Source: CAD feature listing. Evaluate the final solid. Frame: model axes, mm. A direction names the side the tool comes from. Round coordinates to 2 decimals unless told otherwise and drop trailing zeros. Order: outer loops, then holes, each group sorted by start corner. A loop starts at its lowest first (then second) coordinate and runs counter-clockwise, first axis right, second up. Notation, with made-up numbers: M 27.25,-34.75 L 63.25,-34.75 A18 ccw 63.25,-6.75 Z; hole C 55.5,-18.5 d8. An arc over 180 degrees is marked long. Answer in a Markdown table with one row per item. Add a question column.
```python
from build123d import *

# Parameters (mm, degrees)
F0_W     = 32
F0_H     = 19
F1_DEPTH = 4
F2_W     = 32
F2_H     = 4
F3_DEPTH = 16
F5_W     = 14
F5_H     = 6.1
F6_DEPTH = 25
F7_R     = 1.85
F8_DEPTH = 2
F9_D     = 3
F10_R    = 4


with BuildPart() as f1:
    # F0 (on Top) → F1 (new body)
    with BuildSketch(Plane.XY):
        Rectangle(F0_W, F0_H)
    extrude(amount=F1_DEPTH)

    # F2 (on face) → F3 (join)
    with BuildSketch(Plane(origin=(0, 0, 0), x_dir=(1, 0, 0), z_dir=(0, 0, -1))):
        with Locations((0, -7.5)):
            Rectangle(F2_W, F2_H)
    extrude(amount=F3_DEPTH)

    # F5 (on face) → F6 (cut)
    with BuildSketch(Plane.XY.offset(4)):
        with Locations((0, 0.95)):
            Rectangle(F5_W, F5_H)
    extrude(amount=-F6_DEPTH, mode=Mode.SUBTRACT)

    # F7 (on face) → F8 (join)
    with BuildSketch(Plane(origin=(0, 0, 0), x_dir=(1, 0, 0), z_dir=(0, 0, -1))):
        with Locations((-12, 2.5)):
            Circle(F7_R)
        with Locations((12, 2.5)):
            Circle(F7_R)
    extrude(amount=F8_DEPTH)

    # F9 (through all)
    with Locations(Plane.XZ.offset(-5.5)):
        with Locations((-9, -9), (9, -9)):
            Hole(F9_D / 2)

    # F10
    f10_edges = [f1.edges().sort_by_distance(p)[0] for p in [
        (16, -9.5, 2),
        (-16, -9.5, 2),
        (-16, 7.5, -16),
        (16, 7.5, -16),
    ]]
    fillet(f10_edges, radius=F10_R)


solid = f1.part
```
(1) Access query for faces 4 (the face through (-7, 1, 2)), 5 (the face through (12, -3, -2)), 6 (the face through (0, -4, 0)). Directions: +Z, -Z, +X, -X, +Y, -Y. A direction counts if a zero-diameter tool reaches every point of the face in a straight line with its end or side. Return the directions, or none.
(2) Cut plane D-D (x = -9). Return loops of the section in (y, z), and give its area (3 significant figures).
(3) Draft query along X for faces 1 (the face through (14.797, 7.472, -14.859)), 2 (the face through (-10.235, -3.056, -0.986)), 3 (the face through (-14.859, -8.297, 2.028)). Return one class per face: +X half, -X half, draft (parallel to the pull), parting line (faces both ways), or undercut.
(4) Pin query (flat end, axial travel): pin 1 (2.5 mm diameter, centred on x = 9, z = -9, fed in from +Y); pin 2 (1.1 mm diameter, centred on x = 12.5, y = -3, fed in from -Z); pin 3 (1 mm diameter, centred on x = -7, z = -7, fed in from -Y); pin 4 (2 mm diameter, centred on x = 5.5, y = -2, fed in from +Z). Return the tip coordinate at first contact, or that it passes through.
(5) Cut plane C-C (y = 1). Return loops of the section in (x, z), and give its area (3 significant figures).
(6) Cut plane A-A (x = 3). Return loops of the section in (y, z).
(7) Line query: line 1 (Z direction, x = 9, y = 8.6); line 2 (X direction, y = -1.25, z = 1); line 3 (Y direction, x = -8, z = -0.25). Output: solid intervals per line, ascending. Write a range as from..to.
(8) Cut plane B-B (z = -9). Return loops of the section in (x, y), and give its area (3 significant figures).
Answer list:
| question | item | result |
|---|---|---|
| 1 | face 4 | +Z, -Z |
| 1 | face 5 | -Z, +X, -X, -Y |
| 1 | face 6 | -Z |
| 2 | outline | M -9.5,0 L 5.5,0 L 5.5,-7.5 L 9.5,-7.5 L 9.5,4 L -9.5,4 Z; M 5.5,-16 L 9.5,-16 L 9.5,-10.5 L 5.5,-10.5 Z |
| 2 | area | 128 mm² |
| 3 | face 1 | +X half |
| 3 | face 2 | undercut |
| 3 | face 3 | -X half |
| 4 | pin 1 | through |
| 4 | pin 2 | z = -2 |
| 4 | pin 3 | y = 5.5 |
| 4 | pin 4 | z = 4 |
| 5 | outline | M -16,0 L -7,0 L -7,4 L -16,4 Z; M 7,0 L 16,0 L 16,4 L 7,4 Z |
| 5 | area | 72.0 mm² |
| 6 | outline | M -9.5,0 L -2.1,0 L -2.1,4 L -9.5,4 Z; M 4,0 L 5.5,0 L 5.5,-16 L 9.5,-16 L 9.5,4 L 4,4 Z |
| 7 | line 1 | -16..-10.5, -7.5..4 |
| 7 | line 2 | -16..-7, 7..16 |
| 7 | line 3 | 5.5..9.5 |
| 8 | outline | M -16,5.5 L -10.5,5.5 L -10.5,9.5 L -16,9.5 Z; M -7.5,5.5 L 7.5,5.5 L 7.5,9.5 L -7.5,9.5 Z; M 10.5,5.5 L 16,5.5 L 16,9.5 L 10.5,9.5 Z |
| 8 | area | 104 mm² |
